```python
from build123d import *

# Parameters (mm, degrees)
F0_R     = 35
F1_DEPTH = 95
F2_T     = -1.5
F3_R     = 35
F4_DEPTH = 1.5


with BuildPart() as f1:
    # F0 (on Top) → F1 (new body)
    with BuildSketch(Plane.XY):
        Circle(F0_R)
    extrude(amount=F1_DEPTH)

    # F2
    f2_openings = [f1.faces().sort_by_distance(p)[0] for p in [
        (0, 0, 95),
    ]]
    offset(amount=F2_T, openings=f2_openings)

    # F3 (on Top) → F4 (join)
    with BuildSketch(Plane.XY):
        Circle(F3_R)
    extrude(amount=F4_DEPTH)


solid = f1.part
```
Verification items for the finished model (mm, model axes). Round coordinates to 2 decimals unless told otherwise and drop trailing zeros. Write each loop counter-clockwise with the first axis right and the second up, starting at its lowest first coordinate (ties: lowest second). Pieces come first, ordered by that corner, then holes. Notation, with made-up numbers: (70, 53.5) - (129, 53.5) arc R16 cw to (129, 74.5) - close; hole circle Ø7 at (11.5, 85.5). An arc over 180 degrees is marked (long way). Answer as a JSON object with one key per item and string values. Group by question number.
Q1. Thickness scan on line 1 (Y direction, x = 0, z = 59); line 2 (Z direction, x = 13, y = 30.5); line 3 (X direction, y = 17, z = 64). Record the ranges inside material, lowest first.
Q2. Section check A-A, the plane x = 0. Enter the section's corners in (y, z).
Q3. Mould release check, pull along X, two halves, no side actions. Record for faces 1 (the flat face through (0, 0, 1.5)), 2 (the cylindrical face through (-7.262, -32.703, 47.596)), 3 (the flat face through (0, -34, 95)), 4 (the cylindrical face through (-28, -21, 47)): released by +X, released by -X, zero draft, split by the parting line, or undercut.
Q4. Go/stop test with flat-tipped pins: pin 1 Ø1 at (y, z) = (12, 33.5) entering from -X; pin 2 Ø1 at (x, z) = (14.5, 23) entering from +Y; pin 3 Ø3 at (x, z) = (-5, 17.5) entering from -Y. Record where each tip stops, or that it passes through.
Q5. Section check C-C, the plane z = 73. Enter the section's corners in (x, y).
Found:
{
 "1": {"line 1": "y = -35 to -33.5, 33.5 to 35", "line 2": "z = 0 to 1.5", "line 3": "x = -30.59 to -28.87, 28.87 to 30.59"},
 "2": {"outline": "(-35, 0) - (35, 0) - (35, 95) - (33.5, 95) - (33.5, 1.5) - (-33.5, 1.5) - (-33.5, 95) - (-35, 95) - close"},
 "3": {"face 1": "undercut", "face 2": "undercut", "face 3": "zero draft", "face 4": "split by the parting line"},
 "4": {"pin 1": "stops at x = -33.06", "pin 2": "stops at y = 32.08", "pin 3": "stops at y = -34.82"},
 "5": {"outline": "circle Ø70 at (0, 0); hole circle Ø67 at (0, 0)"}
}
